The listing builds one solid part. Answer for the finished solid, in the listing's coordinates (mm). Face numbers are marked on the shaded views. Give positions to 0.01 mm unless a question says otherwise; leave off trailing zeros. Loops run counter-clockwise (first coordinate to the right, second up) from the corner with the lowest first, then second, coordinate; pieces in that order, holes last.
Item 1: Section A-A, the plane y = 972 is taken. Give the vertices of the cut face in (x, z).
Item 2: Consider line 1 along Y through (x, z) = (-294.5, 233.5); line 2 along Y through (x, z) = (-119.5, 227); line 3 along X through (y, z) = (641, 217). Determine where each line is inside the solid, lowest interval first.
Item 3: Section C-C, the plane z = 273 is taken. Give the vertices of the cut face in (x, y), and give its area (3 significant figures).
Item 4: Section D-D, the plane y = 565 is taken. Give the vertices of the cut face in (x, z).
Item 5: The mould has two halves that part along X. Classify the marked faces 1 and 2: pulls with the +X half, pulls with the -X half, needs draft (parallel to the pull), parting line crosses it, or undercut.
Item 6: Section B-B, the plane x = -104 is taken. Give the vertices of the cut face in (y, z), and give its area (3 significant figures).
Item 7: Each of these flat-tipped pins is pushed along its axis until it touches: pin 1 Ø20 at (x, y) = (-7.5, 710.5) entering from +Z; pin 2 Ø15 at (x, y) = (-142, 1105.5) entering from -Z; pin 3 Ø1.5 at (x, y) = (-137, 641.5) entering from -Z; pin 4 Ø12.5 at (y, z) = (511, 243) entering from +X. Where does it stop, or does it pass through?
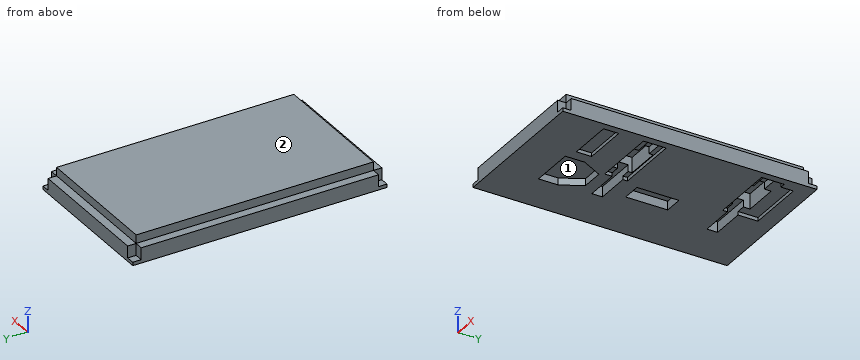
from build123d import *

# Parameters (mm, degrees)
BOX160_W                  = 26
BOX160_H                  = 26
BOX160_DEPTH              = 61
BOX161_W                  = 26
BOX161_H                  = 26
BOX161_DEPTH              = 61
BOX162_W                  = 26
BOX162_H                  = 26
BOX162_DEPTH              = 61
BOX163_W                  = 26
BOX163_H                  = 26
BOX163_DEPTH              = 61
BOX164_W                  = 26
BOX164_H                  = 26
BOX164_DEPTH              = 442
BOX165_W                  = 26
BOX165_H                  = 26
BOX165_DEPTH              = 442
BOX166_W                  = 26
BOX166_H                  = 26
BOX166_DEPTH              = 752
BOX167_W                  = 26
BOX167_H                  = 26
BOX167_DEPTH              = 752
FUSION056_PLACEMENT_ANGLE = 180
BOX129_W                  = 247
BOX129_H                  = 133
BOX129_DEPTH              = 45
BOX123_W                  = 205
BOX123_H                  = 131
BOX123_DEPTH              = 119
BOX123_ROLL_ANGLE         = 118
BOX123_PLACEMENT_ANGLE    = 180
BOX122_W                  = 187
BOX122_H                  = 131
BOX122_DEPTH              = 119
BOX099_W                  = 222
BOX099_H                  = 190
BOX099_DEPTH              = 67
BOX100_W                  = 247
BOX100_H                  = 290
BOX100_DEPTH              = 31.5
BOX098_W                  = 267
BOX098_H                  = 103
BOX098_DEPTH              = 63
BOX128_W                  = 222
BOX128_H                  = 174
BOX128_DEPTH              = 55
BOX114_W                  = 222
BOX114_H                  = 190
BOX114_DEPTH              = 67
BOX115_W                  = 247
BOX115_H                  = 290
BOX115_DEPTH              = 31.5
BOX113_W                  = 267
BOX113_H                  = 103
BOX113_DEPTH              = 63
BOX120_W                  = 237
BOX120_H                  = 55
BOX120_DEPTH              = 124
BOX130_W                  = 750
BOX130_H                  = 70
BOX130_DEPTH              = 440
CUT025_PLACEMENT_ANGLE    = 90


with BuildPart() as cube120:
    # Box160 → Box160 (new body)
    with BuildSketch(Plane(origin=(238, -256, -232), x_dir=(0, 0, 1), z_dir=(-1, 0, 0))):
        with Locations((13, 13)):
            Rectangle(BOX160_W, BOX160_H)
    extrude(amount=BOX160_DEPTH)


with BuildPart() as cube121:
    # Box161 → Box161 (new body)
    with BuildSketch(Plane(origin=(238, -256, 210), x_dir=(0, 1, 0), z_dir=(-1, 0, 0))):
        with Locations((13, 13)):
            Rectangle(BOX161_W, BOX161_H)
    extrude(amount=BOX161_DEPTH)


with BuildPart() as cube122:
    # Box162 → Box162 (new body)
    with BuildSketch(Plane(origin=(238, 496, -232), x_dir=(0, -1, 0), z_dir=(-1, 0, 0))):
        with Locations((13, 13)):
            Rectangle(BOX162_W, BOX162_H)
    extrude(amount=BOX162_DEPTH)


with BuildPart() as cube123:
    # Box163 → Box163 (new body)
    with BuildSketch(Plane(origin=(238, 496, 210), x_dir=(0, 0, -1), z_dir=(-1, 0, 0))):
        with Locations((13, 13)):
            Rectangle(BOX163_W, BOX163_H)
    extrude(amount=BOX163_DEPTH)


with BuildPart() as cube124:
    # Box164 → Box164 (new body)
    with BuildSketch(Plane(origin=(238, 496, 210), x_dir=(0, -1, 0), z_dir=(0, 0, -1))):
        with Locations((13, 13)):
            Rectangle(BOX164_W, BOX164_H)
    extrude(amount=BOX164_DEPTH)


with BuildPart() as cube125:
    # Box165 → Box165 (new body)
    with BuildSketch(Plane(origin=(238, -230, 210), x_dir=(0, -1, 0), z_dir=(0, 0, -1))):
        with Locations((13, 13)):
            Rectangle(BOX165_W, BOX165_H)
    extrude(amount=BOX165_DEPTH)


with BuildPart() as cube126:
    # Box166 → Box166 (new body)
    with BuildSketch(Plane(origin=(238, 496, 210), x_dir=(-1, 0, 0), z_dir=(0, -1, 0))):
        with Locations((13, 13)):
            Rectangle(BOX166_W, BOX166_H)
    extrude(amount=BOX166_DEPTH)


with BuildPart() as supportbeams001:
    # Box167 → Box167 (new body)
    with BuildSketch(Plane(origin=(238, 496, -206), x_dir=(-1, 0, 0), z_dir=(0, -1, 0))):
        with Locations((13, 13)):
            Rectangle(BOX167_W, BOX167_H)
    extrude(amount=BOX167_DEPTH)

    # Fusion056: union Cube120, Cube121, Cube122, Cube123, Cube124, Cube125, Cube126
    add(cube120.part)
    add(cube121.part)
    add(cube122.part)
    add(cube123.part)
    add(cube124.part)
    add(cube125.part)
    add(cube126.part)


with BuildPart() as supportbeams001_1:
    # Fusion056 placement: moved
    add(supportbeams001.part.moved(Location((172, 240, 0))).rotate(Axis((172, 240, 0), (0, 0, 1)), FUSION056_PLACEMENT_ANGLE))


with BuildPart() as f_120_envelope007:
    # Box129 → Box129 (new body)
    with BuildSketch(Plane(origin=(241.570357, -122, 54.646476), x_dir=(-1, 0, 0), z_dir=(0, 1, 0))):
        with Locations((123.5, 66.5)):
            Rectangle(BOX129_W, BOX129_H)
    extrude(amount=BOX129_DEPTH)


with BuildPart() as pocket009:
    # Box123 → Box123 (new body)
    with BuildSketch(Plane.XY):
        with Locations((102.5, 65.5)):
            Rectangle(BOX123_W, BOX123_H)
    extrude(amount=BOX123_DEPTH)


with BuildPart() as pocket009_1:
    # Box123 roll: moved
    add(pocket009.part.rotate(Axis((0, 0, 0), (1, 0, 0)), BOX123_ROLL_ANGLE))


with BuildPart() as pocket009_2:
    # Box123 placement: moved
    add(pocket009_1.part.moved(Location((141.57, -85, 25.646476))).rotate(Axis((141.57, -85, 25.646476), (0, 0, 1)), BOX123_PLACEMENT_ANGLE))


with BuildPart() as compound014:
    # Part__Mirroring003: instance of pocket009
    add(pocket009_2.part.mirror(Plane(origin=(0, 0, 0), x_dir=(0, 1, 0), z_dir=(0, 0, 1))))


with BuildPart() as compound014_1:
    # Compound014 placement: moved
    add(compound014.part.moved(Location((0, 0, -88))))


with BuildPart() as fusion043:
    # Fusion043 base: copy of pocket009
    add(pocket009_2.part)

    # Fusion043: union Compound014
    add(compound014_1.part)


with BuildPart() as prism002:
    # Box122 → Box122 (new body)
    with BuildSketch(Plane(origin=(136.57, -135, -109.353524), x_dir=(-1, 0, 0), z_dir=(0, 1, 0))):
        with Locations((93.5, 65.5)):
            Rectangle(BOX122_W, BOX122_H)
    extrude(amount=BOX122_DEPTH)

    # Cut020: cut Fusion043
    add(fusion043.part, mode=Mode.SUBTRACT)


with BuildPart() as prism002_1:
    # Cut020 placement: moved
    add(prism002.part.moved(Location((35, 0, 0))))


with BuildPart() as cube073:
    # Box099 → Box099 (new body)
    with BuildSketch(Plane(origin=(216.570357, -4, -2.353524), x_dir=(-1, 0, 0), z_dir=(0, 1, 0))):
        with Locations((111, 95)):
            Rectangle(BOX099_W, BOX099_H)
    extrude(amount=BOX099_DEPTH)


with BuildPart() as cube074:
    # Box100 → Box100 (new body)
    with BuildSketch(Plane(origin=(221.570357, 18, -102.353524), x_dir=(-1, 0, 0), z_dir=(0, 1, 0))):
        with Locations((123.5, 145)):
            Rectangle(BOX100_W, BOX100_H)
    extrude(amount=BOX100_DEPTH)


with BuildPart() as standard_envelope002:
    # Box098 → Box098 (new body)
    with BuildSketch(Plane(origin=(216.570357, -2, 23.646476), x_dir=(-1, 0, 0), z_dir=(0, 1, 0))):
        with Locations((133.5, 51.5)):
            Rectangle(BOX098_W, BOX098_H)
    extrude(amount=BOX098_DEPTH)

    # Fusion036: union Cube073, Cube074
    add(cube073.part)
    add(cube074.part)


with BuildPart() as obj1:
    # Box128 → Box128 (new body)
    with BuildSketch(Plane(origin=(216.570357, 393, -2.353524), x_dir=(-1, 0, 0), z_dir=(0, 1, 0))):
        with Locations((111, 87)):
            Rectangle(BOX128_W, BOX128_H)
    extrude(amount=BOX128_DEPTH)


with BuildPart() as cube088:
    # Box114 → Box114 (new body)
    with BuildSketch(Plane(origin=(216.570357, -4, -2.353524), x_dir=(-1, 0, 0), z_dir=(0, 1, 0))):
        with Locations((111, 95)):
            Rectangle(BOX114_W, BOX114_H)
    extrude(amount=BOX114_DEPTH)


with BuildPart() as cube089:
    # Box115 → Box115 (new body)
    with BuildSketch(Plane(origin=(221.570357, 18, -102.353524), x_dir=(-1, 0, 0), z_dir=(0, 1, 0))):
        with Locations((123.5, 145)):
            Rectangle(BOX115_W, BOX115_H)
    extrude(amount=BOX115_DEPTH)


with BuildPart() as standard_envelope003:
    # Box113 → Box113 (new body)
    with BuildSketch(Plane(origin=(216.570357, -2, 23.646476), x_dir=(-1, 0, 0), z_dir=(0, 1, 0))):
        with Locations((133.5, 51.5)):
            Rectangle(BOX113_W, BOX113_H)
    extrude(amount=BOX113_DEPTH)

    # Fusion042: union Cube088, Cube089
    add(cube088.part)
    add(cube089.part)


with BuildPart() as fusion053:
    # Part__Mirroring002: instance of Standard envelope003
    add(standard_envelope003.part.mirror(Plane(origin=(0, 0, 0), x_dir=(1, 0, 0), z_dir=(0, 1, 0))))


with BuildPart() as fusion053_1:
    # Part__Mirroring002 placement: moved
    add(fusion053.part.moved(Location((0, 407.25, 0))))

    # Fusion053: union obj1
    add(obj1.part)


with BuildPart() as fusion054:
    # Box120 → Box120 (new body)
    with BuildSketch(Plane(origin=(216.570357, 100, -72.353524), x_dir=(-1, 0, 0), z_dir=(0, 1, 0))):
        with Locations((118.5, 27.5)):
            Rectangle(BOX120_W, BOX120_H)
    extrude(amount=BOX120_DEPTH)

    # Fusion054: union 120 envelope007, prism002, Standard envelope002, Fusion053
    add(f_120_envelope007.part)
    add(prism002_1.part)
    add(standard_envelope002.part)
    add(fusion053_1.part)


with BuildPart() as cut025:
    # Box130 → Box130 (new body)
    with BuildSketch(Plane(origin=(5, -255, -231), x_dir=(0, 1, 0), z_dir=(0, 0, 1))):
        with Locations((375, 35)):
            Rectangle(BOX130_W, BOX130_H)
    extrude(amount=BOX130_DEPTH)

    # Cut024: cut Fusion054
    add(fusion054.part, mode=Mode.SUBTRACT)

    # Cut025: cut Supportbeams001
    add(supportbeams001_1.part, mode=Mode.SUBTRACT)


with BuildPart() as cut025_1:
    # Cut025 placement: moved
    add(cut025.part.moved(Location((-204, 755, 215))).rotate(Axis((-204, 755, 215), (0, 1, 0)), CUT025_PLACEMENT_ANGLE))


solid = cut025_1.part
Worked answers:
1. outline: (-435, 210) - (-276.35, 210) - (-276.35, 235.43) - (-221.35, 235.43) - (-221.35, 210) - (5, 210) - (5, 255) - (-20, 255) - (-20, 280) - (-410, 280) - (-410, 255) - (-435, 255) - close
2. line 1: y = 500 to 773, 804.5 to 1112.75, 1144.25 to 1250
2. line 2: y = 500 to 753, 816 to 1101.25, 1164.25 to 1250
2. line 3: x = -435 to -313.35, -182.35 to -149.35, -16.35 to 5
3. outline: (-410, 525) - (-20, 525) - (-20, 1225) - (-410, 1225) - close
3. area: 273,000 mm2
4. outline: (-435, 210) - (5, 210) - (5, 255) - (-20, 255) - (-20, 280) - (-410, 280) - (-410, 255) - (-435, 255) - close
5. face 1: undercut
5. face 2: needs draft
6. outline: (500, 210) - (633, 210) - (633, 220.43) - (678, 220.43) - (678, 210) - (751, 210) - (751, 220.43) - (753, 220.43) - (753, 265.43) - (816, 265.43) - (816, 220.43) - (818, 220.43) - (818, 210) - (1099.25, 210) - (1099.25, 220.43) - (1101.25, 220.43) - (1101.25, 265.43) - (1164.25, 265.43) - (1164.25, 220.43) - (1203, 220.43) - (1203, 210) - (1250, 210) - (1250, 255) - (1225, 255) - (1225, 280) - (525, 280) - (525, 255) - (500, 255) - close
6. area: 43,300 mm2
7. pin 1: stops at z = 255
7. pin 2: stops at z = 210
7. pin 3: stops at z = 220.43
7. pin 4: stops at x = -20
